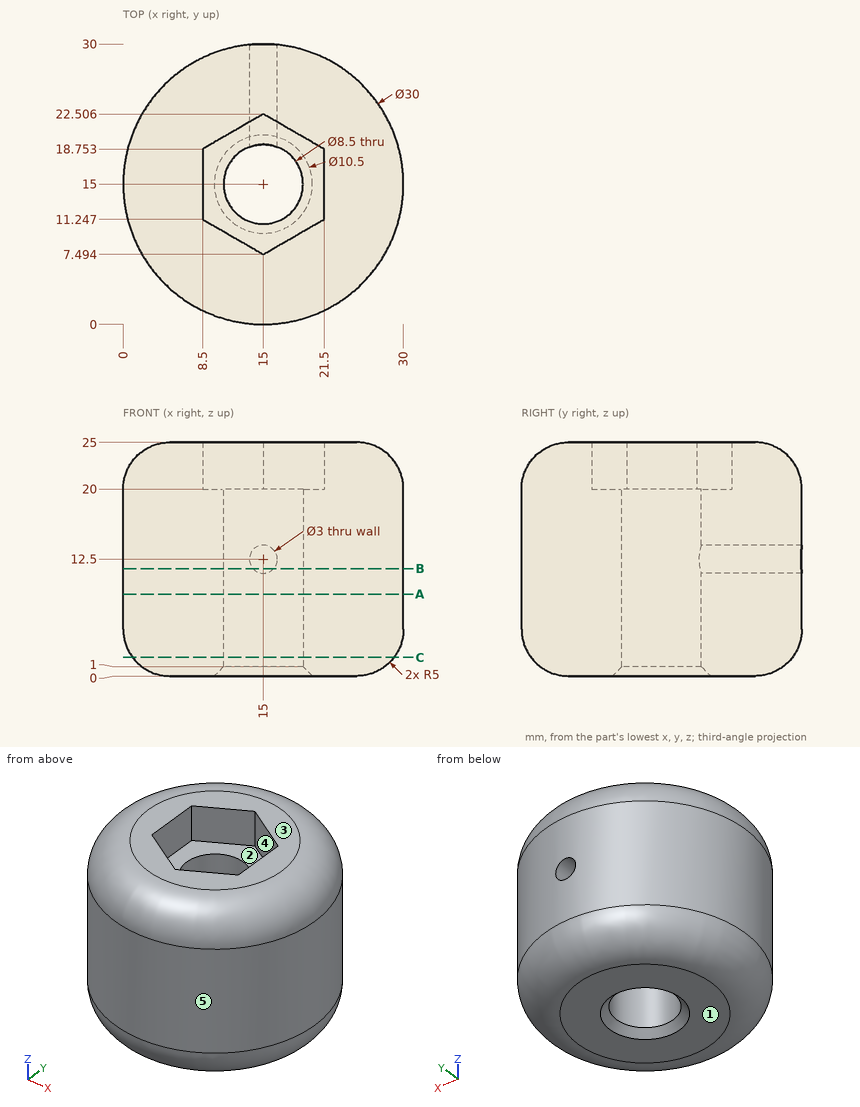
Design review of the part shown in the three views and the two pictorial views. Dimensions are in mm from the part's minimum x, y and z. A direction names the side the tool comes from. Give positions to 0.01 mm unless a question says otherwise; leave off trailing zeros. Loops run counter-clockwise (first coordinate to the right, second up) from the corner with the lowest first, then second, coordinate; pieces in that order, holes last. Notation, with made-up numbers: (-22.5, -35) - (-3.5, -35) arc R14 cw to (-3.5, -10) - close; hole circle Ø8 at (-26, 12). An arc over 180 degrees is marked (long way). Answer as a JSON object with one key per item and string values.
Q1. Add section B-B on z = 11.5. State the section outline as (x, y) points.
Worked out:
{"outline": "(13.88, 19.1) - (13.88, 29.96) arc R15 ccw (long way) to (16.12, 29.96) - (16.12, 19.1) arc R4.25 cw (long way) to start"}
Q2. Insertion check: pin 1 (2.5 mm diameter, centred on x = 15, z = 12.5, fed in from +Y); pin 2 (10 mm diameter, centred on y = 22, z = 9, fed in from -X). Each pin has a flat end and moves straight along its axis. Give the tip position at first contact, or say it passes through.
Worked out:
{"pin 1": "stops at y = 10.94", "pin 2": "stops at x = 0.13"}
Q3. Mouldability with a two-part tool opening along X and no side actions: class the marked faces 3, 4 and 5 as +X half, -X half, draft (parallel to the pull), parting line (faces both ways), or undercut.
Worked out:
{"face 3": "draft", "face 4": "undercut", "face 5": "parting line"}
Q4. To check wall thickness, follow line 1 along Y through (x, z) = (15, 9.25); line 2 along X through (y, z) = (18, 11.25) (1 decimal); line 3 along Z through (x, y) = (20.5, 12.5). State the ranges of each line that lie inside material, in increasing order.
Worked out:
{"line 1": "y = 0 to 10.75, 19.25 to 30", "line 2": "x = 0.3 to 12, 18 to 29.7", "line 3": "z = 0 to 20"}
Q5. Add section C-C on z = 2. State the section outline as (x, y) points.
Worked out:
{"outline": "circle Ø28 at (15, 15); hole circle Ø8.5 at (15, 15)"}
Q6. For the marked faces 1 and 2, list the 3-axis set-ups (+Z, -Z, +X, -X, +Y, -Y) from which the entire face can be reached by the end or side of a thin tool; tool diameter is ignored.
Worked out:
{"face 1": "-Z, +X, -X, +Y, -Y", "face 2": "+Z"}
Q7. Add section A-A on z = 8.75. State the section outline as (x, y) points.
Worked out:
{"outline": "circle Ø30 at (15, 15); hole circle Ø8.5 at (15, 15)"}
